from build123d import *

# Parameters (mm, degrees)
SKETCH_1_R          = 30
EXTRUDE_1_DEPTH     = 1
SKETCH_10_R         = 30
SKETCH_10_R_2       = 28
EXTRUDE_4_DEPTH     = 10
SKETCH_11_W         = 8.5
SKETCH_11_H         = 8.5
EXTRUDE_5_DEPTH     = 3
EXTRUDE_START       = 29
SKETCH_17_R         = 4.571283513
EXTRUDE_6_DEPTH     = 2
SKETCH_18_W         = 4.174244664
SKETCH_18_H         = 6.326589568
CUT_EXTRUDE_5_DEPTH = 10
SKETCH_19_R         = 30
SKETCH_19_R_2       = 25
EXTRUDE_7_DEPTH     = 1
SKETCH_23_R         = 30
SKETCH_23_R_2       = 26
EXTRUDE_8_DEPTH     = 1.5
CUT_EXTRUDE_START   = -2
SKETCH_24_R         = 32
SKETCH_24_R_2       = 28
CUT_EXTRUDE_6_DEPTH = 2
EXTRUDE_START_2     = 4
SKETCH_25_R         = 30
EXTRUDE_9_DEPTH     = 4
SKETCH_26_R         = 1.5
CUT_EXTRUDE_7_DEPTH = 4
EXTRUDE_START_3     = 5
SKETCH_27_R         = 29.5
SKETCH_27_R_2       = 1.5
EXTRUDE_10_DEPTH    = 5


with BuildPart() as part:
    # 草图1 → 凸台-拉伸1 (new body)
    with BuildSketch(Plane(origin=(0, 0, 0), x_dir=(1, 0, 0), z_dir=(0, 1, 0))):
        with Locations(Location((0, 0, 0), (0, 0, 270))):
            Circle(SKETCH_1_R)
    extrude(amount=EXTRUDE_1_DEPTH)

    # 草图10 → 凸台-拉伸4 (add)
    with BuildSketch(Plane(origin=(0, 1, 0), x_dir=(1, 0, 0), z_dir=(0, 1, 0))):
        with Locations(Location((0, 0, 0), (0, 0, 270))):
            Circle(SKETCH_10_R)
        with Locations(Location((0, 0, 0), (0, 0, 270))):
            Circle(SKETCH_10_R_2, mode=Mode.SUBTRACT)
    extrude(amount=EXTRUDE_4_DEPTH)

    # 草图11 → 凸台-拉伸5 (add)
    with BuildSketch(Plane(origin=(0, 1, 0), x_dir=(1, 0, 0), z_dir=(0, 1, 0))):
        Rectangle(SKETCH_11_W, SKETCH_11_H)
    extrude(amount=EXTRUDE_5_DEPTH)

    # 草图17 → 凸台-拉伸6 (add)
    with BuildSketch(Plane.XY.offset(EXTRUDE_START)):
        with Locations(Location((0, 4.876571378, 0), (0, 0, 180))):
            Circle(SKETCH_17_R)
    extrude(amount=EXTRUDE_6_DEPTH)

    # 草图18 → 切除-拉伸5 (cut)
    with BuildSketch(Plane.XY.offset(31)):
        with Locations((0, 4.876571378)):
            Rectangle(SKETCH_18_W, SKETCH_18_H)
    extrude(amount=-CUT_EXTRUDE_5_DEPTH, mode=Mode.SUBTRACT)

    # 草图19 → 凸台-拉伸7 (add)
    with BuildSketch(Plane(origin=(0, 11, 0), x_dir=(1, 0, 0), z_dir=(0, 1, 0))):
        with Locations(Location((0, 0, 0), (0, 0, 270))):
            Circle(SKETCH_19_R)
        with Locations(Location((0, 0, 0), (0, 0, 270))):
            Circle(SKETCH_19_R_2, mode=Mode.SUBTRACT)
    extrude(amount=EXTRUDE_7_DEPTH)

    # 草图23 → 凸台-拉伸8 (add)
    with BuildSketch(Plane(origin=(0, 12, 0), x_dir=(1, 0, 0), z_dir=(0, 1, 0))):
        with Locations(Location((0, 0, 0), (0, 0, 270))):
            Circle(SKETCH_23_R)
        with Locations(Location((0, 0, 0), (0, 0, 270))):
            Circle(SKETCH_23_R_2, mode=Mode.SUBTRACT)
    extrude(amount=EXTRUDE_8_DEPTH)

    # 草图24 → 切除-拉伸6 (cut)
    with BuildSketch(Plane(origin=(0, 13.5, 0), x_dir=(1, 0, 0), z_dir=(0, 1, 0)).offset(CUT_EXTRUDE_START)):
        Circle(SKETCH_24_R)
        with Locations(Location((0, 0, 0), (0, 0, 270))):
            Circle(SKETCH_24_R_2, mode=Mode.SUBTRACT)
    extrude(amount=CUT_EXTRUDE_6_DEPTH, mode=Mode.SUBTRACT)

    # 草图25 → 凸台-拉伸9 (add)
    with BuildSketch(Plane.XZ.offset(EXTRUDE_START_2)):
        with Locations(Location((0, 0, 0), (0, 0, 270))):
            Circle(SKETCH_25_R)
    extrude(amount=-EXTRUDE_9_DEPTH)

    # 草图26 → 切除-拉伸7 (cut)
    with BuildSketch(Plane(origin=(0, -4, 0), x_dir=(-1, 0, 0), z_dir=(0, -1, 0))):
        with Locations(Location((-10.25961511, 17.034507364, 0), (0, 0, 90))):
            Circle(SKETCH_26_R)
        with Locations(Location((10.74038489, 17.034507364, 0), (0, 0, 270))):
            Circle(SKETCH_26_R)
        with Locations(Location((10.74038489, -16.965492636, 0), (0, 0, 90))):
            Circle(SKETCH_26_R)
        with Locations(Location((-10.25961511, -16.965492636, 0), (0, 0, 270))):
            Circle(SKETCH_26_R)
    extrude(amount=-CUT_EXTRUDE_7_DEPTH, mode=Mode.SUBTRACT)

    # 草图27 → 凸台-拉伸10 (add)
    with BuildSketch(Plane.XZ.offset(4).offset(EXTRUDE_START_3)):
        with Locations(Location((0, 0, 0), (0, 0, 270))):
            Circle(SKETCH_27_R)
        with Locations(Location((-10.74038489, 16.965492636, 0), (0, 0, 270))):
            Circle(SKETCH_27_R_2, mode=Mode.SUBTRACT)
        with Locations(Location((-10.74038489, -17.034507364, 0), (0, 0, 270))):
            Circle(SKETCH_27_R_2, mode=Mode.SUBTRACT)
        with Locations(Location((10.25961511, -17.034507364, 0), (0, 0, 270))):
            Circle(SKETCH_27_R_2, mode=Mode.SUBTRACT)
        with Locations(Location((10.25961511, 16.965492636, 0), (0, 0, 270))):
            Circle(SKETCH_27_R_2, mode=Mode.SUBTRACT)
    extrude(amount=-EXTRUDE_10_DEPTH)


solid = part.part
Could you check a few things on this model? Use its own coordinates, in mm. A direction names the side the tool comes from. Give positions to 0.01 mm unless a question says otherwise; leave off trailing zeros. Order: outer loops, then holes, each group sorted by start corner. A loop starts at its lowest first (then second) coordinate and runs counter-clockwise, first axis right, second up.
1. Suppose I cut it at A-A (z = 0). List the corners of the cut face in (x, y) for me, plus the area to 4 significant figures.
2. For faces 1 (the flat face through (10, 0, 17)), 2 (the cylindrical face through (-15.821, 12.74, -20.633)), 3 (the flat face through (0, 1.713, 29)), which set-ups out of +Z, -Z, +X, -X, +Y, -Y let a thin tool reach every point of the face, with its end or its side?
3. I need wall thicknesses on L1, parallel to Y at x = -22, z = 15; L2, parallel to X at y = -3.75, z = -17; L3, parallel to Z at x = -11, y = 12.5. Which ranges of each line are inside material? Lowest first, please.
4. We'd pull the mould along X, two halves only. Please class faces 4 (the cylindrical face through (8.86, -6.54, -28.14)), 5 (the flat face through (3, 5, 31)), 6 (the flat face through (0, 1, 6)), 7 (the flat face through (-11, 0, -17)): pulls with the +X half, pulls with the -X half, needs draft (parallel to the pull), parting line crosses it, or undercut.
5. Will these pins go through, and if not, where does the flat tip stop? P1, Ø6, axis at x = -5.5, y = -6, coming from the +Z side; P2, Ø0.9, axis at x = -1, z = 30, coming from the -Y side; P3, Ø8, axis at x = 0, z = -10.5, coming from the +Y side.
6. Suppose I cut it at B-B (x = -22.5). List the corners of the cut face in (y, z) for me, plus the area to 3 significant figures.
7. Suppose I cut it at C-C (y = 5.75). List the corners of the cut face in (x, z) for me.
8. Suppose I cut it at D-D (y = -2). List the corners of the cut face in (x, z) for me.
Solved:
1. outline: (-30, -4) - (-29.5, -4) - (-29.5, -9) - (29.5, -9) - (29.5, -4) - (30, -4) - (30, 11.5) - (28, 11.5) - (28, 13.5) - (26, 13.5) - (26, 12) - (25, 12) - (25, 11) - (28, 11) - (28, 1) - (4.25, 1) - (4.25, 4) - (-4.25, 4) - (-4.25, 1) - (-28, 1) - (-28, 11) - (-25, 11) - (-25, 12) - (-26, 12) - (-26, 13.5) - (-28, 13.5) - (-28, 11.5) - (-30, 11.5) - close
1. area: 674.5 mm2
2. face 1: -Y
2. face 2: +Y
2. face 3: +Z
3. L1: y = -9 to 1, 11 to 13.5
3. L2: x = -24.72 to -12.24, -9.24 to 8.76, 11.76 to 24.72
3. L3: z = -25.75 to -23.56, 23.56 to 25.75
4. face 4: parting line crosses it
4. face 5: needs draft
4. face 6: undercut
4. face 7: undercut
5. P1: stops at z = 29.82
5. P2: stops at y = -4
5. P3: stops at y = 1
6. outline: (-9, -19.08) - (-4, -19.08) - (-4, -19.84) - (11.5, -19.84) - (11.5, -16.67) - (13.5, -16.67) - (13.5, -13.03) - (12, -13.03) - (12, -10.9) - (11, -10.9) - (11, -16.67) - (1, -16.67) - (1, 16.67) - (11, 16.67) - (11, 10.9) - (12, 10.9) - (12, 13.03) - (13.5, 13.03) - (13.5, 16.67) - (11.5, 16.67) - (11.5, 19.84) - (-4, 19.84) - (-4, 19.08) - (-9, 19.08) - close
6. area: 478 mm2
7. outline: (-4.49, 29.66) arc R30 ccw (long way) to (4.49, 29.66) - (4.49, 31) - (2.09, 31) - (2.09, 27.92) arc R28 cw (long way) to (-2.09, 27.92) - (-2.09, 31) - (-4.49, 31) - close
8. outline: circle Ø60 at (0, 0); hole circle Ø3 at (-10.74, -17.03); hole circle Ø3 at (-10.74, 16.97); hole circle Ø3 at (10.26, -17.03); hole circle Ø3 at (10.26, 16.97)
